from build123d import *

# Parameters (mm, degrees)
F0_R     = 1.5875
F1_DEPTH = 76.2


with BuildPart() as f1:
    # F0 (on Front) → F1 (new body)
    with BuildSketch(Plane.XZ):
        with BuildLine():
            ThreePointArc((36.357702, 11.389799), (40.273671, 9.510209), (42.417319, 13.288099))
            ThreePointArc((42.417319, 13.288099), (42.346482, 13.512141), (42.274462, 13.735805))
            ThreePointArc((42.274462, 13.735805), (0, 44.45), (-42.274462, 13.735805))
            ThreePointArc((-42.274462, 13.735805), (-42.346482, 13.512141), (-42.417319, 13.288099))
            ThreePointArc((-42.417319, 13.288099), (-40.273671, 9.510209), (-36.357702, 11.389799))
            ThreePointArc((-36.357702, 11.389799), (-36.296985, 11.581835), (-36.235253, 11.773547))
            ThreePointArc((-36.235253, 11.773547), (0, 38.1), (36.235253, 11.773547))
            ThreePointArc((36.235253, 11.773547), (36.296985, 11.581835), (36.357702, 11.389799))
        make_face()
        with Locations((-39.254858, 12.754676)):
            Circle(F0_R, mode=Mode.SUBTRACT)
        with Locations((39.254858, 12.754676)):
            Circle(F0_R, mode=Mode.SUBTRACT)
        with Locations((-12.754676, 39.254858)):
            Circle(F0_R, mode=Mode.SUBTRACT)
        with Locations((12.754676, 39.254858)):
            Circle(F0_R, mode=Mode.SUBTRACT)
        with BuildLine():
            ThreePointArc((42.274462, 13.735805), (42.346482, 13.512141), (42.417319, 13.288099))
            ThreePointArc((42.417319, 13.288099), (42.354166, 13.514593), (42.274462, 13.735805))
        make_face()
        with BuildLine():
            ThreePointArc((36.235253, 11.773547), (36.2904, 11.579734), (36.357702, 11.389799))
            ThreePointArc((36.357702, 11.389799), (36.296985, 11.581835), (36.235253, 11.773547))
        make_face()
        with BuildLine():
            ThreePointArc((-42.417319, 13.288099), (-42.346482, 13.512141), (-42.274462, 13.735805))
            ThreePointArc((-42.274462, 13.735805), (-42.354166, 13.514593), (-42.417319, 13.288099))
        make_face()
        with BuildLine():
            ThreePointArc((-36.357702, 11.389799), (-36.2904, 11.579734), (-36.235253, 11.773547))
            ThreePointArc((-36.235253, 11.773547), (-36.296985, 11.581835), (-36.357702, 11.389799))
        make_face()
    extrude(amount=F1_DEPTH)


solid = f1.part
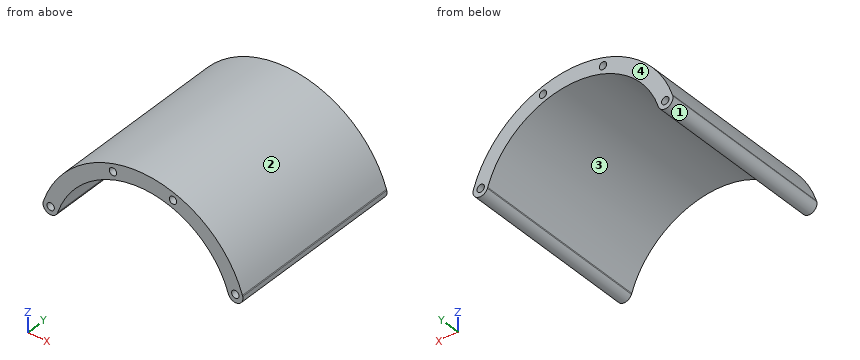
Could you check a few things on this model? Use its own coordinates, in mm. Face numbers are marked on the shaded views. Round coordinates to 2 decimals unless told otherwise and drop trailing zeros. Loops run counter-clockwise (first coordinate to the right, second up) from the corner with the lowest first, then second, coordinate; pieces in that order, holes last. Notation, with made-up numbers: (-11.5, -30) - (27.5, -30) arc R22 ccw to (27.5, -4) - close; hole circle Ø2 at (7, -15). An arc over 180 degrees is marked (long way). Write item = value, one per line.
1) I need wall thicknesses on line 1 along X through (y, z) = (-65.5, 39.5); line 2 along Z through (x, y) = (1, -57.5); line 3 along X through (y, z) = (-65, 18). Which ranges of each line are inside material? Lowest first, please. Write a range as from..to.
Computed:
line_1 = -20.39..-14.32, -11.19..11.19, 14.32..20.39
line_2 = 38.09..44.44
line_3 = -40.64..-33.58, 33.58..40.64
2) If we mould it in two halves opening along X, with no side actions, what happens to the marked faces 1, 2, 3 and 4? For each: pulls with the +X half, pulls with the -X half, needs draft (parallel to the pull), parting line crosses it, or undercut.
Computed:
face_1 = undercut
face_2 = parting line crosses it
face_3 = undercut
face_4 = needs draft
3) Imagine slicing it at C-C (z = 16). Please give me the cut outline in (x, y), and give its area (3 significant figures).
Computed:
outline = (-41.47, -76.2) - (-34.58, -76.2) - (-34.58, 0) - (-41.47, 0) - close; (34.58, -76.2) - (41.47, -76.2) - (41.47, 0) - (34.58, 0) - close
area = 1,050 mm2
4) I'm going to push flat-ended pins straight in: P1, Ø2.5, axis at x = -39.25, z = 12.75, coming from the +Y side; P2, Ø2, axis at y = -55.5, z = 19, coming from the +X side; P3, Ø6, axis at y = -45, z = 36, coming from the -X side; P4, Ø3, axis at y = -35.5, z = 37, coming from the -X side. Where does each tip first touch, or does it pass through?
Computed:
P1 = through
P2 = 40.64
P3 = -29.78
P4 = -26.75
5) Imagine slicing it at D-D (x = 17). Please give me the cut outline in (y, z), and give its area (3 significant figures).
Computed:
outline = (-76.2, 34.1) - (0, 34.1) - (0, 41.07) - (-76.2, 41.07) - close
area = 531 mm2
6) Imagine slicing it at A-A (z = 25). Please give me the cut outline in (x, y), and give its area (3 significant figures).
Computed:
outline = (-36.75, -76.2) - (-28.75, -76.2) - (-28.75, 0) - (-36.75, 0) - close; (28.75, -76.2) - (36.75, -76.2) - (36.75, 0) - (28.75, 0) - close
area = 1,220 mm2
7) Imagine slicing it at B-B (y = -53.5). Give the number of separate pieces and of enclosed holes in the cut face, and give its area (3 significant figures).
Computed:
separate_pieces = 1
enclosed_holes = 4
area = 662 mm2
